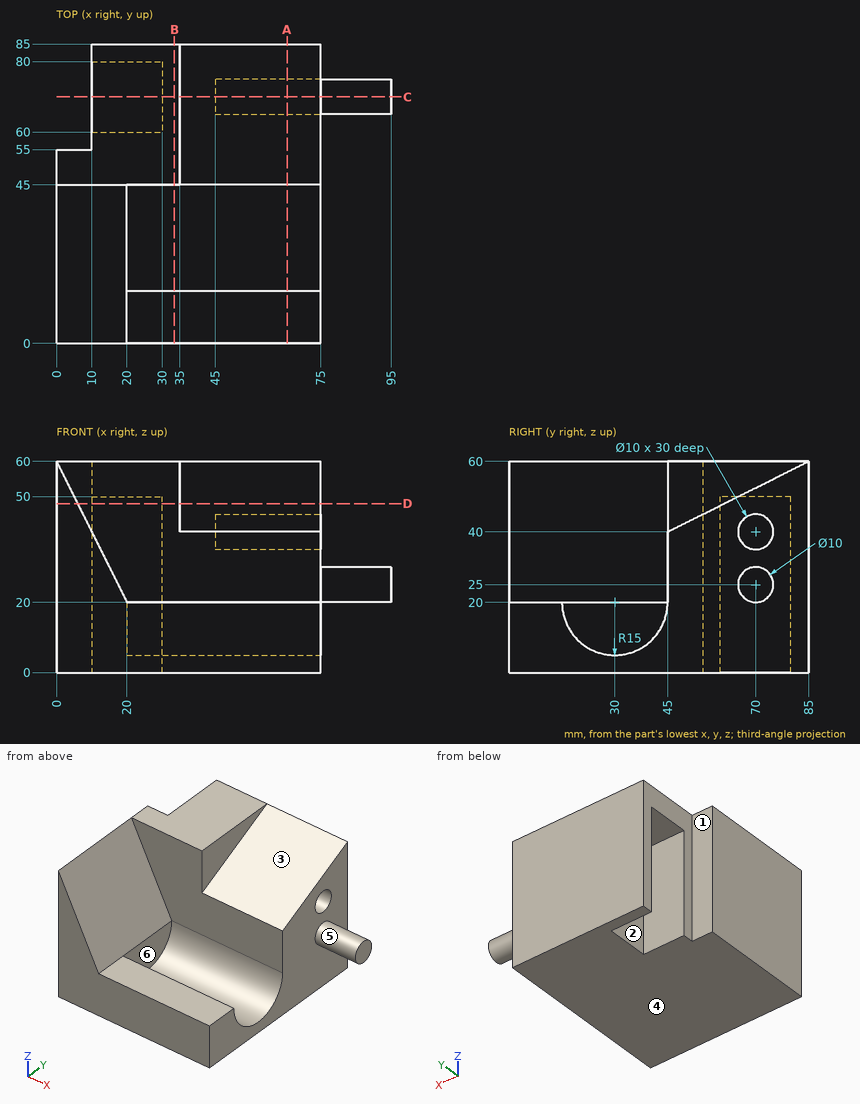
Study the drawing (mm; zero at the part's minimum x, y, z) and answer. A direction names the side the tool comes from. Give positions to 0.01 mm unless a question says otherwise; leave off trailing zeros. Loops run counter-clockwise (first coordinate to the right, second up) from the corner with the lowest first, then second, coordinate; pieces in that order, holes last. Notation, with made-up numbers: M 54,-34.5 L 99,-34.5 A33 ccw 99,1.5 Z; hole C 85.25,67 d2. An arc over 180 degrees is marked long. One line per item, written item: value. Start each with the question number.
1. Find section D-D (z = 48). Give the vertices of the cut face in (x, y).
2. Find section C-C (y = 70). Give the vertices of the cut face in (x, z), and give its area (3 significant figures).
3. Each of these flat-tipped pins is pushed along its axis until it touches: P1, Ø5, axis at y = 42, z = 28.5, coming from the +X side; P2, Ø9, axis at y = 70, z = 40, coming from the +X side; P3, Ø22, axis at y = 71, z = 26.5, coming from the -X side. Where does it stop, or does it pass through?
4. Find section B-B (x = 33.5). Give the vertices of the cut face in (y, z).
5. Which of the six approach directions +Z, -Z, +X, -X, +Y, -Y give full straight-line access (tool end or side, diameter ignored) to the marked faces 1, 2 and 3?
6. Find section A-A (x = 65.5). Give the vertices of the cut face in (y, z), and give its area (3 significant figures).
7. Determine the mould class of the marked faces 4, 5 and 6 for opening direction Y: released by +Y, released by -Y, zero draft, split by the parting line, or undercut.
8. Find the intervals of material crossed by probe 1 along X at (y, z) = (63.5, 16.5); probe 2 along Z at (x, y) = (60.25, 70); probe 3 along Z at (x, y) = (66, 10), in increasing order.
Reported:
1. outline: M 0,0 L 6,0 L 6,45 L 35,45 L 35,61 L 75,61 L 75,85 L 10,85 L 10,80 L 30,80 L 30,60 L 10,60 L 10,55 L 0,55 Z
2. outline: M 10,50 L 30,50 L 30,0 L 75,0 L 75,20 L 95,20 L 95,30 L 75,30 L 75,35 L 45,35 L 45,45 L 75,45 L 75,52.5 L 35,52.5 L 35,60 L 10,60 Z
2. area: 2,500 mm²
3. P1: stops at x = 17
3. P2: stops at x = 45
3. P3: stops at x = 10
4. outline: M 0,0 L 85,0 L 85,60 L 45,60 L 45,20 A15 cw 15,20 L 0,20 Z
5. face 1: +Z, -Z, -X, +Y
5. face 2: -Z, -X
5. face 3: +Z, +X, -Y
6. outline: M 0,0 L 85,0 L 85,60 L 45,40 L 45,20 A15 cw 15,20 L 0,20 Z; hole C 70,40 d10
6. area: 2,470 mm²
7. face 4: zero draft
7. face 5: split by the parting line
7. face 6: undercut
8. probe 1: x = 30 to 75
8. probe 2: z = 0 to 35, 45 to 52.5
8. probe 3: z = 0 to 20
